Work out the finished part from the listing and answer in its coordinate system (mm). Face numbers are marked on the shaded views. A direction names the side the tool comes from. Round coordinates to 2 decimals unless told otherwise and drop trailing zeros. Write each loop counter-clockwise with the first axis right and the second up, starting at its lowest first coordinate (ties: lowest second). Pieces come first, ordered by that corner, then holes.
1. A tool of negligible diameter and unlimited length cuts with its end or side. For the marked faces 4, 5 and 6, from which of +Z, -Z, +X, -X, +Y, -Y can it reach the whole face along a straight path? Write none if from no direction.
2. Determine the mould class of the marked faces 1, 2 and 3 for opening direction Y: pulls with the +Y half, pulls with the -Y half, needs draft (parallel to the pull), parting line crosses it, or undercut.
3. Find section A-A (x = 0). Write down the section's boundary in (y, z), and give its area (3 significant figures).
4. Straight lines are drawn through the part: probe 1 along Y at (x, z) = (0, 4.25); probe 2 along Y at (x, z) = (0, 6.75); probe 3 along X at (y, z) = (1.75, 0.75). For each, find the intervals that lie inside material, in ascending order.
5. Find section D-D (z = 1). Write down the section's boundary in (x, y).
6. Flat-ended cylindrical pins translate along their axes: pin 1 Ø4 at (y, z) = (-2, 0.5) entering from +X; pin 2 Ø3 at (x, z) = (-2, 3) entering from -Y; pin 3 Ø4 at (x, y) = (1, 0.5) entering from +Z. Find the tip coordinate at first contact, or state that the pin passes through.
7. Find section C-C (z = 6.25). Write down the section's boundary in (x, y).
```python
from build123d import *

# Parameters (mm, degrees)
SKETCH1_R           = 3.9
SKETCH1_R_2         = 2.65
BOSS_EXTRUDE1_DEPTH = 5
BOSS_EXTRUDE2_START = -2
SKETCH2_R           = 6
SKETCH2_R_2         = 2.65
BOSS_EXTRUDE2_DEPTH = 2
BOSS_EXTRUDE3_START = 2
SKETCH3_R           = 3.9
BOSS_EXTRUDE3_DEPTH = 2
FILLET1_R           = 1
SKETCH4_R           = 3.85
SKETCH4_R_2         = 2.65
BOSS_EXTRUDE4_DEPTH = 4


with BuildPart() as part:
    # Sketch1 → Boss-Extrude1 (new body)
    with BuildSketch(Plane.XY):
        Circle(SKETCH1_R)
        Circle(SKETCH1_R_2, mode=Mode.SUBTRACT)
    extrude(amount=BOSS_EXTRUDE1_DEPTH)

    # Sketch2 → Boss-Extrude2 (add)
    with BuildSketch(Plane.XY.offset(5).offset(BOSS_EXTRUDE2_START)):
        Circle(SKETCH2_R)
        Circle(SKETCH2_R_2, mode=Mode.SUBTRACT)
    extrude(amount=BOSS_EXTRUDE2_DEPTH)

    # Sketch3 → Boss-Extrude3 (add)
    with BuildSketch(Plane(origin=(0, 0, 0), x_dir=(-1, 0, 0), z_dir=(0, 0, -1)).offset(BOSS_EXTRUDE3_START)):
        Circle(SKETCH3_R)
    extrude(amount=-BOSS_EXTRUDE3_DEPTH)

    # Fillet1
    fillet1_edges = [part.edges().sort_by_distance(p)[0] for p in [
        (3.9, 0, -2),
    ]]
    fillet(fillet1_edges, radius=FILLET1_R)

    # Sketch4 → Boss-Extrude4 (add)
    with BuildSketch(Plane.XY.offset(5)):
        Circle(SKETCH4_R)
        Circle(SKETCH4_R_2, mode=Mode.SUBTRACT)
    extrude(amount=BOSS_EXTRUDE4_DEPTH)


solid = part.part
```
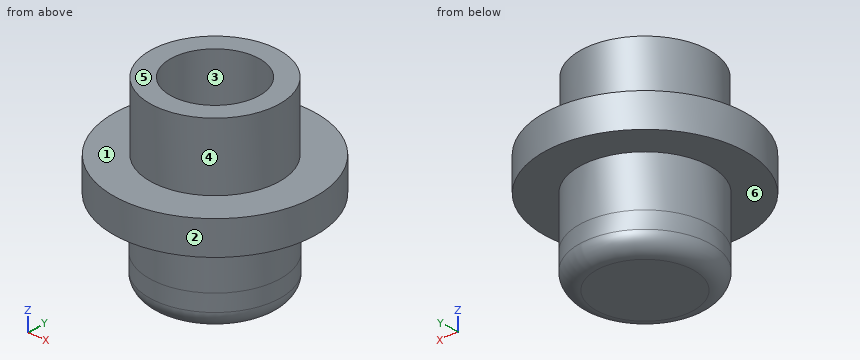
Worked answers:
1. face 4: +Z
1. face 5: +Z, +X, -X, +Y, -Y
1. face 6: -Z
2. face 1: needs draft
2. face 2: parting line crosses it
2. face 3: undercut
3. outline: (-6, 3) - (-3.9, 3) - (-3.9, -1) arc R1 ccw to (-2.9, -2) - (2.9, -2) arc R1 ccw to (3.9, -1) - (3.9, 3) - (6, 3) - (6, 5) - (3.85, 5) - (3.85, 9) - (2.65, 9) - (2.65, 0) - (-2.65, 0) - (-2.65, 9) - (-3.85, 9) - (-3.85, 5) - (-6, 5) - close
3. area: 45.7 mm2
4. probe 1: y = -6 to -2.65, 2.65 to 6
4. probe 2: y = -3.85 to -2.65, 2.65 to 3.85
4. probe 3: x = -3.49 to -1.99, 1.99 to 3.49
5. outline: circle Ø7.8 at (0, 0); hole circle Ø5.3 at (0, 0)
6. pin 1: stops at x = 3.9
6. pin 2: stops at y = -5.98
6. pin 3: stops at z = 9
7. outline: circle Ø7.7 at (0, 0); hole circle Ø5.3 at (0, 0)
